Check sheet for the drawn part. Datum: minimum x, y, z corner. Units: mm. Coordinates: 2 decimals unless noted, no trailing zeros. Write each loop counter-clockwise with the first axis right and the second up, starting at its lowest first coordinate (ties: lowest second). Pieces come first, ordered by that corner, then holes. Notation, with made-up numbers: (43.5, 64.25) -> (87.5, 64.25) arc R25 ccw to (87.5, 82.25) -> close; hole circle Ø5 at (-28.75, 69.5). An arc over 180 degrees is marked (long way). Answer in a Markdown table with one row per item. Add a question column.
Q1. Thickness scan on line 1 (Z direction, x = 75, y = 6.5); line 2 (X direction, y = 4.5, z = 45); line 3 (X direction, y = 9.75, z = 51). Record the ranges inside material, lowest first.
Q2. Section check B-B, the plane x = 75. Record the boundary of the cut face in (y, z), and give its area (3 significant figures).
Q3. Section check A-A, the plane z = 45. Record the boundary of the cut face in (x, y), and give its area (3 significant figures).
Q4. Section check C-C, the plane y = 5.75. Record the boundary of the cut face in (x, z), and give its area (3 significant figures).
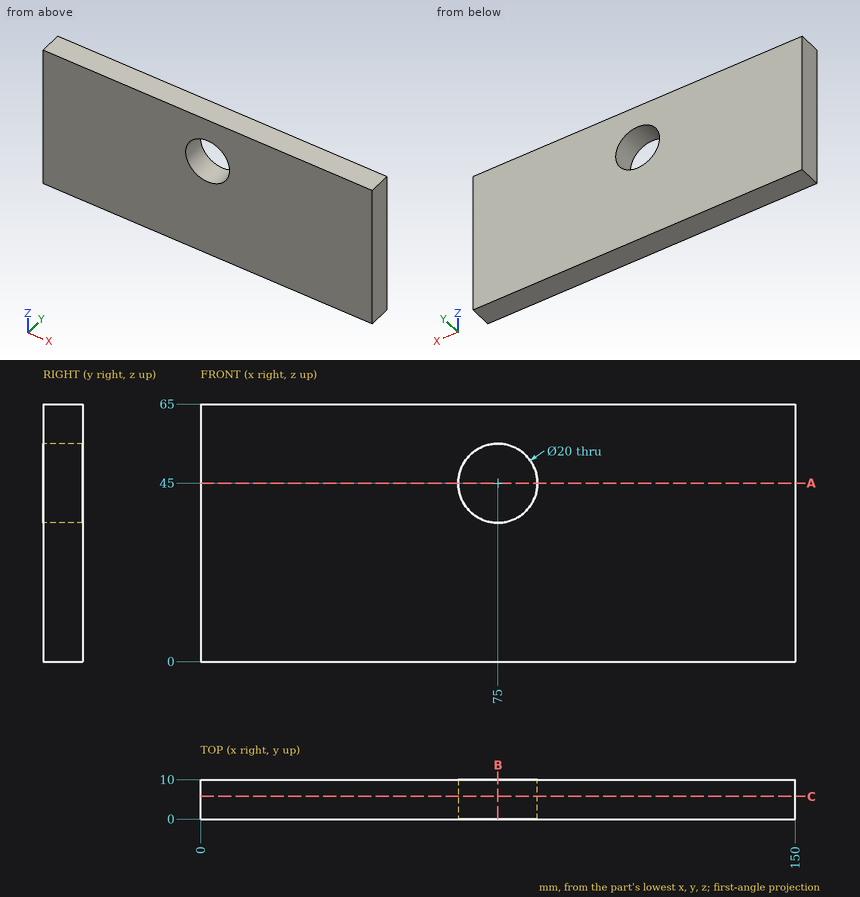
Calculated:
| question | item | result |
|---|---|---|
| 1 | line 1 | z = 0 to 35, 55 to 65 |
| 1 | line 2 | x = 0 to 65, 85 to 150 |
| 1 | line 3 | x = 0 to 67, 83 to 150 |
| 2 | outline | (0, 0) -> (10, 0) -> (10, 35) -> (0, 35) -> close; (0, 55) -> (10, 55) -> (10, 65) -> (0, 65) -> close |
| 2 | area | 450 mm² |
| 3 | outline | (0, 0) -> (65, 0) -> (65, 10) -> (0, 10) -> close; (85, 0) -> (150, 0) -> (150, 10) -> (85, 10) -> close |
| 3 | area | 1,300 mm² |
| 4 | outline | (0, 0) -> (150, 0) -> (150, 65) -> (0, 65) -> close; hole circle Ø20 at (75, 45) |
| 4 | area | 9,440 mm² |
